from build123d import *

# Parameters (mm, degrees)
F0_R     = 3.175
F1_DEPTH = 153
F2_W     = 21.5
F2_H     = 75
F2_W_2   = 23.88
F2_H_2   = 65.41
F3_DEPTH = 12.5


with BuildPart() as f1:
    # F0 (on Top) → F1 (new body)
    with BuildSketch(Plane.XY):
        with BuildLine():
            Line((-16.601021, -1), (16.601021, -1))
            ThreePointArc((16.601021, -1), (26.5, 0), (16.601021, 1))
            Line((16.601021, 1), (-16.601021, 1))
            ThreePointArc((-16.601021, 1), (-26.5, 0), (-16.601021, -1))
        make_face()
        with Locations((-21.5, 0)):
            Circle(F0_R, mode=Mode.SUBTRACT)
        with Locations((21.5, 0)):
            Circle(F0_R, mode=Mode.SUBTRACT)
    extrude(amount=F1_DEPTH)

    # F2 (on Front) → F3 (cut, symmetric)
    with BuildSketch(Plane.XZ):
        with Locations((0, 37.5)):
            Rectangle(F2_W, F2_H)
        with Locations((0.08833, 118.608861)):
            Rectangle(F2_W_2, F2_H_2)
    extrude(amount=F3_DEPTH, both=True, mode=Mode.SUBTRACT)


solid = f1.part
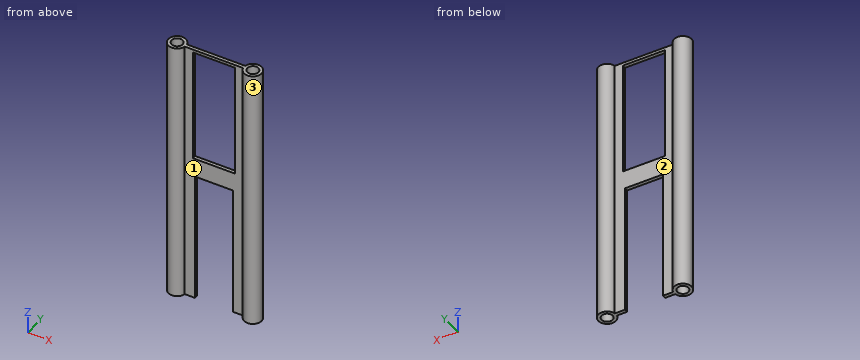
Work out the finished part from the listing and answer in its coordinate system (mm). Face numbers are marked on the shaded views. A direction names the side the tool comes from. Coordinates: 2 decimals unless noted, no trailing zeros. Write each loop counter-clockwise with the first axis right and the second up, starting at its lowest first coordinate (ties: lowest second). Pieces come first, ordered by that corner, then holes. Notation, with made-up numbers: M -39,19 L 16,19 A32 cw 16,54 Z; hole C -27,18 d7. An arc over 180 degrees is marked long. Answer as CSV lines item,"result". Start each with the question number.
Item 1: Section C-C on z = 93 is taken. Write down the section's boundary in (x, y) (3 decimals).
Item 2: Consider L1, parallel to X at y = 0.25, z = 101.5; L2, parallel to Y at x = -21.5, z = 82 (3 decimals); L3, parallel to X at y = 2.5, z = 46.5. Determine where each line is inside the solid, lowest interval first.
Item 3: Section D-D on x = 8.5 is taken. Write down the section's boundary in (y, z), and give its area (3 significant figures).
Item 4: Section B-B on x = 21.5 is taken. Write down the section's boundary in (y, z) (3 decimals), and give its area (3 significant figures).
Item 5: A tool of negligible diameter and unlimited length cuts with its end or side. For the marked faces 1, 2 and 3, from which of +Z, -Z, +X, -X, +Y, -Y can it reach the whole face along a straight path? Write none if from no direction.
Item 6: Section A-A on z = 27 is taken. Write down the section's boundary in (x, y) (3 decimals), and give its area (3 significant figures).
Item 7: Flat-ended cylindrical pins translate along their axes: P1, Ø3, axis at y = -2.5, z = 32.5, coming from the -X side; P2, Ø2, axis at x = 5, y = -0.5, coming from the -Z side; P3, Ø10, axis at x = 8, z = 71, coming from the -Y side; P4, Ø8, axis at x = 7.5, z = 132.5, coming from the +Y side. Find the tip coordinate at first contact, or state that the pin passes through.
Checks:
1,outline,"M -16.601,-1 L -11.852,-1 L -11.852,1 L -16.601,1 A5 ccw long Z; M 12.028,-1 L 16.601,-1 A5 ccw long 16.601,1 L 12.028,1 Z; hole C -21.5,0 d6.35; hole C 21.5,0 d6.35"
2,L1,"x = -26.49 to -24.67, -18.33 to -11.85, 12.03 to 18.33, 24.67 to 26.49"
2,L2,"y = -5 to -3.175, 3.175 to 5"
2,L3,"x = -25.83 to -23.46, -19.54 to -17.17, 17.17 to 19.54, 23.46 to 25.83"
3,outline,"M -1,75 L 1,75 L 1,85.9 L -1,85.9 Z; M -1,151.31 L 1,151.31 L 1,153 L -1,153 Z"
3,area,"25.2 mm²"
4,outline,"M -5,0 L -3.175,0 L -3.175,153 L -5,153 Z; M 3.175,0 L 5,0 L 5,153 L 3.175,153 Z"
4,area,"558 mm²"
5,face 1,"+Z, -Z, -Y"
5,face 2,"+Z, -Z, +Y"
5,face 3,"+Z, -Z"
6,outline,"M -16.601,-1 L -10.75,-1 L -10.75,1 L -16.601,1 A5 ccw long Z; M 10.75,-1 L 16.601,-1 A5 ccw long 16.601,1 L 10.75,1 Z; hole C -21.5,0 d6.35; hole C 21.5,0 d6.35"
6,area,"117 mm²"
7,P1,"stops at x = -26.4"
7,P2,"stops at z = 75"
7,P3,"stops at y = -1"
7,P4,"passes through"
